Input: dimensioned drawing with shaded views. Units: mm. Origin: part minimum x, y, z. Give positions to 0.01 mm unless a question says otherwise; leave off trailing zeros. Write each loop counter-clockwise with the first axis right and the second up, starting at its lowest first coordinate (ties: lowest second). Pieces come first, ordered by that corner, then holes. Notation, with made-up numbers: M -35,33.5 L 10,33.5 A6 ccw 10,37.5 Z; hole C 82.25,56 d8. An arc over 180 degrees is marked long. Answer as a JSON object with one key per item and string values.
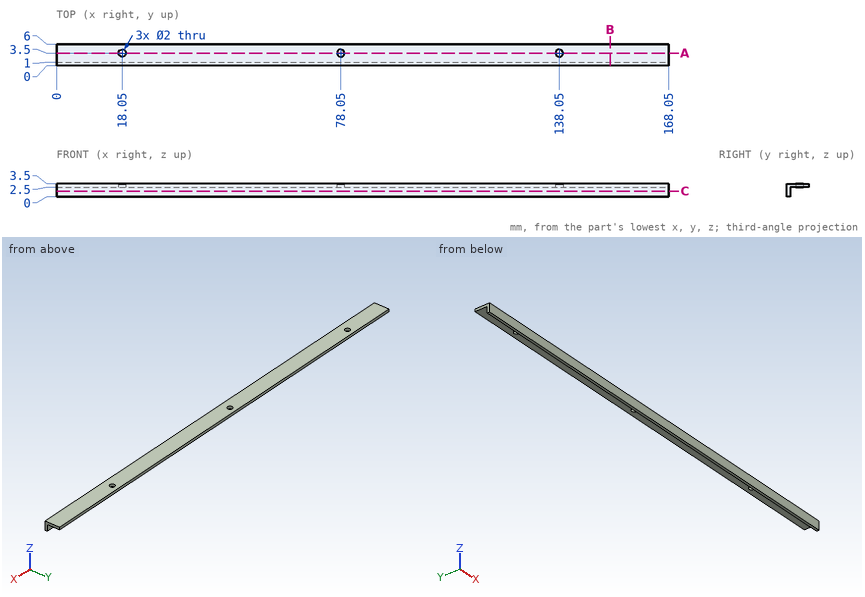
1) Cut plane C-C on z = 1.5. Return loops of the section in (x, y), and give its area (3 significant figures).
Geometry check:
{"outline": "M 0,0 L 168.05,0 L 168.05,1 L 0,1 Z", "area": "168 mm2"}
2) Line query: line 1 (X direction, y = 4.3, z = 3); line 2 (Y direction, x = 138.05, z = 2.9); line 3 (Z direction, x = 88, y = 2.7). Output: solid intervals per line, ascending. Write a range as from..to.
Geometry check:
{"line 1": "x = 0..17.45, 18.65..77.45, 78.65..137.45, 138.65..168.05", "line 2": "y = 0..2.5, 4.5..6", "line 3": "z = 2.5..3.5"}
3) Cut plane A-A on y = 3.5. Return loops of the section in (x, z), and give its area (3 significant figures).
Geometry check:
{"outline": "M 0,2.5 L 17.05,2.5 L 17.05,3.5 L 0,3.5 Z; M 19.05,2.5 L 77.05,2.5 L 77.05,3.5 L 19.05,3.5 Z; M 79.05,2.5 L 137.05,2.5 L 137.05,3.5 L 79.05,3.5 Z; M 139.05,2.5 L 168.05,2.5 L 168.05,3.5 L 139.05,3.5 Z", "area": "162 mm2"}
4) Contact query for flat-ended pins moving along their axis: P1, Ø1, axis at x = 120.5, z = 0.5, coming from the +Y side; P2, Ø2.5, axis at x = 78.05, y = 3.5, coming from the -Z side; P3, Ø2, axis at x = 146.5, z = 2.5, coming from the -Y side. Output: stop coordinate, or through.
Geometry check:
{"P1": "stops at y = 1", "P2": "stops at z = 2.5", "P3": "stops at y = 0"}
5) Cut plane B-B on x = 152. Return loops of the section in (y, z).
Geometry check:
{"outline": "M 0,0 L 1,0 L 1,2.5 L 6,2.5 L 6,3.5 L 0,3.5 Z"}
